Autodesk Fusion 360 part; units mm, degrees
sketch "Skizze1" plane through (0, 0, 0) normal (0, 0, 1) x (1, 0, 0)
  line L0 (258, 143.5) -> (0, 143.5)
  circle A0 centre (229, 39.5) radius 2.25
  circle A1 centre (229, 21.5) radius 2.25
  circle A2 centre (59, 54) radius 1.5
  circle A3 centre (4.5, 4.5) radius 1.5
  circle A4 centre (222, 54) radius 1.5
  circle A5 centre (4.5, 139) radius 1.5
  circle A6 centre (253.5, 4.5) radius 1.5
  circle A7 centre (253.5, 139) radius 1.5
  circle A8 centre (124.5, 4.5) radius 1.5
  circle A9 centre (253.5, 71.75) radius 1.5
  line L1 (0, 143.5) -> (0, 0)
  circle A10 centre (59, 39.5) radius 2.25
  circle A11 centre (20, 4.5) radius 1.5
  circle A12 centre (229, 4.5) radius 1.5
  circle A13 centre (59, 21.5) radius 2.25
  circle A14 centre (4.5, 71.75) radius 1.5
  line L2 (0, 143.5) -> (0, 0) construction
  line L3 (9, 143.5) -> (0, 143.5) construction
  circle A15 centre (133, 54) radius 1.5
  line L4 (0, 0) -> (258, 0)
  line L5 (0, 0) -> (9, 0) construction
  line L6 (258, 0) -> (258, 143.5)
  circle A16 centre (173.1, 134.4) radius 2.25
  arc A17 (210.3507, 143.5) -> (207.6493, 143.5) centre (209, 98.5) ccw construction
  arc A18 (249, 119.1597) -> (229.6597, 138.5) centre (209, 98.5) ccw
  arc A19 (188.3403, 138.5) -> (170.2508, 121.4199) centre (209, 98.5) ccw
  arc A20 (170.2508, 75.5801) -> (188.3403, 58.5) centre (209, 98.5) ccw
  arc A21 (229.6597, 58.5) -> (249, 77.8403) centre (209, 98.5) ccw
  circle A22 centre (244.9, 134.4) radius 2.25
  circle A23 centre (173.1, 62.6) radius 2.25
  circle A24 centre (244.9, 62.6) radius 2.25
  line L7 (188.3403, 138.5) -> (229.6597, 138.5)
  line L8 (249, 119.1597) -> (249, 77.8403)
  line L9 (188.3403, 58.5) -> (229.6597, 58.5)
  arc A25 (149.6597, 58.5) -> (167.7492, 75.5801) centre (129, 98.5) ccw
  arc A26 (167.7492, 121.4199) -> (149.6597, 138.5) centre (129, 98.5) ccw
  line L10 (108.3403, 138.5) -> (149.6597, 138.5)
  arc A27 (108.3403, 138.5) -> (89, 119.1597) centre (129, 98.5) ccw
  line L11 (89, 119.1597) -> (89, 77.8403)
  arc A28 (89, 77.8403) -> (108.3403, 58.5) centre (129, 98.5) ccw
  line L12 (108.3403, 58.5) -> (149.6597, 58.5)
  circle A29 centre (93.1, 134.4) radius 2.25
  circle A30 centre (93.1, 62.6) radius 2.25
  circle A31 centre (164.9, 62.6) radius 2.25
  circle A32 centre (164.9, 134.4) radius 2.25
  arc A33 (167.7492, 121.4199) -> (170.2508, 121.4199) centre (169, 122.1597) ccw
  arc A34 (170.2508, 75.5801) -> (167.7492, 75.5801) centre (169, 74.8403) ccw
  point P0 (253.5, 71.75)
  point P1 (253.5, 139)
  point P2 (253.5, 4.5)
  point P3 (253.5, 4.5)
  point P4 (253.5, 139)
  point P5 (253.5, 71.75)
  dimension "d1" = 143.5
  dimension "d2" = 258
  dimension "d6" = 18
  dimension "d7" = 4.5
  dimension "d8" = 4.5
  dimension "d9" = 4.5
  dimension "d10" = 4.5
  dimension "d11" = 3
  dimension "d12" = 3
  dimension "d13" = 3
  dimension "d14" = 3
  dimension "d15" = 3
  dimension "d22" = 20
  dimension "d24" = 209
  dimension "d26" = 104.5
  dimension "d27" = 3
  dimension "d28" = 3
  dimension "d29" = 3
  dimension "d30" = 67.25
  dimension "d31" = 9
  dimension "d32" = 67.25
  dimension "d33" = 67.25
  dimension "d34" = 3
  dimension "d35" = 3
  dimension "d36" = 3
  dimension "d37" = 67.25
  dimension "d45" = 2.25
  dimension "d47" = 4.5
  dimension "d48" = 4.5
  dimension "d49" = 4.5
  dimension "d50" = 2.25
  dimension "d51" = 4.5
  dimension "d52" = 4.5
  dimension "d53" = 4.5
extrude "Extrusion1" add sketch "Skizze1" along normal blind 9
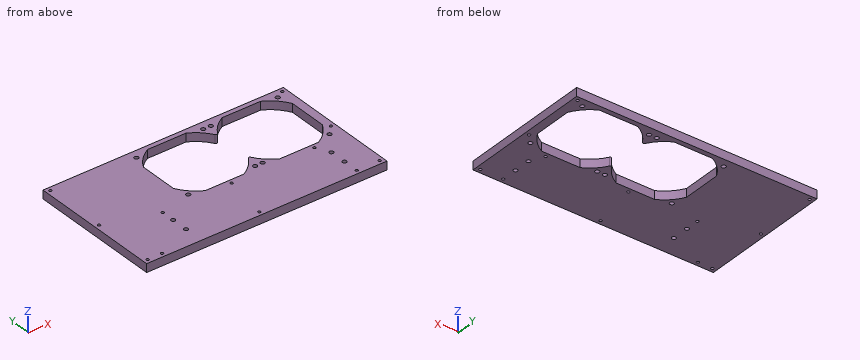
For this review, take the finished solid that the model builds, in its own axes (mm). Give positions to 0.01 mm unless a question says otherwise; leave off trailing zeros. Write each loop counter-clockwise with the first axis right and the second up, starting at its lowest first coordinate (ties: lowest second). Pieces come first, ordered by that corner, then holes. Notation, with made-up numbers: M 1,61.5 L 11,61.5 A10 ccw 11,69.5 Z; hole C -15.5,9 d11. An arc over 180 degrees is marked long. Answer as a JSON object with one key per item and string values. Group by question number.
Item 1: For probe 1 along Y at (x, z) = (4.5, 3.75); probe 2 along X at (y, z) = (111, 4.5); probe 3 along X at (y, z) = (71.75, 6.75), list the stretches that pass through material, from the lowest coordinate up. Write a range as [from, to].
Item 2: Consider section A-A on x = 204. Write out the cut boundary in (y, z).
Item 3: Consider section B-B on z = 1.75. Count the separate pieces of the cut face and the enclosed holes in it, plus the area to 3 significant figures.
Check result:
{
 "1": {"probe 1": "y = [0, 3], [6, 70.25], [73.25, 137.5], [140.5, 143.5]", "probe 2": "x = [0, 89], [249, 258]", "probe 3": "x = [0, 3], [6, 92.79], [165.21, 172.79], [245.21, 252], [255, 258]"},
 "2": {"outline": "M 0,0 L 58.5,0 L 58.5,9 L 0,9 Z; M 138.5,0 L 143.5,0 L 143.5,9 L 138.5,9 Z"},
 "3": {"separate pieces": "1", "enclosed holes": "25", "area": "25,100 mm^2"}
}
